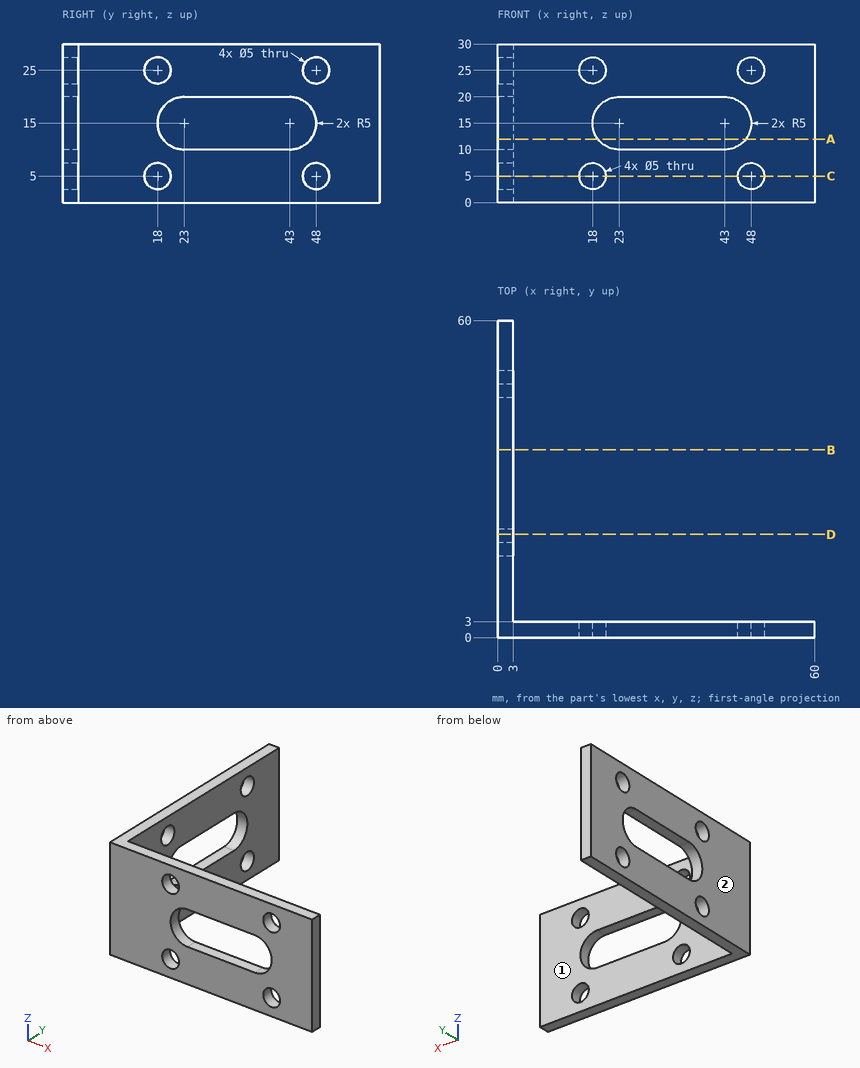
For this review, use the dimensioned drawing (mm, ordinates from the lowest corner) and the shaded views. A direction names the side the tool comes from. Give positions to 0.01 mm unless a question says otherwise; leave off trailing zeros. Order: outer loops, then holes, each group sorted by start corner. A loop starts at its lowest first (then second) coordinate and runs counter-clockwise, first axis right, second up.
1) Take a section at A-A (z = 12). Give the boundary of the cut face in (x, y).
2) Insertion check: pin 1 (2 mm diameter, centred on y = 9.5, z = 5.5, fed in from +X); pin 2 (3 mm diameter, centred on x = 48, z = 25, fed in from +Y); pin 3 (3.5 mm diameter, centred on x = 1, y = 29, fed in from -Z); pin 4 (6.5 mm diameter, centred on x = 18, z = 5, fed in from +Y). Each pin has a flat end and moves straight along its axis. Give the tip position at first contact, or say it passes through.
3) Take a section at B-B (y = 35.5). Give the boundary of the cut face in (x, z), then the cut area to 3 significant figures.
4) Take a section at C-C (z = 5). Give the boundary of the cut face in (x, y).
5) Take a section at D-D (y = 19.5). Give the boundary of the cut face in (x, z).
6) For the marked faces 1 and 2, list the 3-axis set-ups (+Z, -Z, +X, -X, +Y, -Y) from which the entire face can be reached by the end or side of a thin tool; tool diameter is ignored.
7) Wall thickness on line 1 (Y direction, x = 2.1, z = 25); line 2 (X direction, y = 37, z = 6.5): over which ranges is each line inside the solid? List them lowest first.
Derived:
1. outline: (0, 0) - (19, 0) - (19, 3) - (3, 3) - (3, 19) - (0, 19) - close; (0, 47) - (3, 47) - (3, 60) - (0, 60) - close; (47, 0) - (60, 0) - (60, 3) - (47, 3) - close
2. pin 1: stops at x = 3
2. pin 2: passes through
2. pin 3: stops at z = 0
2. pin 4: stops at y = 3
3. outline: (0, 0) - (3, 0) - (3, 10) - (0, 10) - close; (0, 20) - (3, 20) - (3, 30) - (0, 30) - close
3. area: 60.0 mm2
4. outline: (0, 0) - (15.5, 0) - (15.5, 3) - (3, 3) - (3, 15.5) - (0, 15.5) - close; (0, 20.5) - (3, 20.5) - (3, 45.5) - (0, 45.5) - close; (0, 50.5) - (3, 50.5) - (3, 60) - (0, 60) - close; (20.5, 0) - (45.5, 0) - (45.5, 3) - (20.5, 3) - close; (50.5, 0) - (60, 0) - (60, 3) - (50.5, 3) - close
5. outline: (0, 0) - (3, 0) - (3, 3) - (0, 3) - close; (0, 7) - (3, 7) - (3, 11.43) - (0, 11.43) - close; (0, 18.57) - (3, 18.57) - (3, 23) - (0, 23) - close; (0, 27) - (3, 27) - (3, 30) - (0, 30) - close
6. face 1: +Z, -Z, +X, +Y
6. face 2: +Z, -Z, -X, +Y, -Y
7. line 1: y = 0 to 15.5, 20.5 to 45.5, 50.5 to 60
7. line 2: x = 0 to 3
